Input: part model. Units: mm. Frame: model coordinates. A direction names the side the tool comes from. Coordinates: 2 decimals unless noted, no trailing zeros. Write each loop counter-clockwise with the first axis right and the second up, starting at its lowest first coordinate (ties: lowest second). Pieces come first, ordered by that corner, then holes. Notation, with made-up numbers: (54, 61) -> (75, 61) arc R30 ccw to (75, 94) -> close; hole circle Ø9 at (43.25, -26.75). An arc over 180 degrees is marked (long way). One line per question, with ' | ' between items. Start each with the question number.
```python
from build123d import *

# Parameters (mm, degrees)
F0_W     = 17
F0_H     = 2.9
F1_DEPTH = 14
F2_W     = 1.625
F2_H     = 0.32
F2_W_2   = 1
F2_H_2   = 0.58
F3_DEPTH = 12.5
F4_W     = 17
F4_H     = 1.6
F5_DEPTH = 2
F6_SIZE  = 1


with BuildPart() as f1:
    # F0 (on Top) → F1 (new body)
    with BuildSketch(Plane.XY):
        with Locations((8.5, 1.45)):
            Rectangle(F0_W, F0_H)
    extrude(amount=F1_DEPTH)

    # F2 (on face) → F3 (cut)
    with BuildSketch(Plane.XY.offset(14)):
        Polygon((15.375, 2.9), (8.5, 2.9), (1.625, 2.9), (1.625, 2.58), (1.625, 1.3), (15.375, 1.3), (15.375, 2.58), align=None)
        with Locations((16.1875, 2.74)):
            Rectangle(F2_W, F2_H)
        with Locations((0.8125, 2.74)):
            Rectangle(F2_W, F2_H)
        with Locations((16.5, 1.59)):
            Rectangle(F2_W_2, F2_H_2)
        with Locations((0.5, 1.59)):
            Rectangle(F2_W_2, F2_H_2)
    extrude(amount=-F3_DEPTH, mode=Mode.SUBTRACT)

    # F4 (on face) → F5 (cut)
    with BuildSketch(Plane.XY.offset(14)):
        with Locations((8.5, 2.1)):
            Rectangle(F4_W, F4_H)
    extrude(amount=-F5_DEPTH, mode=Mode.SUBTRACT)

    # F6
    f6_edges = [f1.edges().sort_by_distance(p)[0] for p in [
        (8.5, 0, 0),
    ]]
    chamfer(f6_edges, length=F6_SIZE)


solid = f1.part
```
1) Section A-A, the plane z = 7.75. Return loops of the section in (x, y) (3 decimals), then the cut area to 3 significant figures.
2) Section C-C, the plane y = 0.35. Return loops of the section in (x, z).
3) Ray query, line 1 (X direction, y = 1.4, z = 8.5) (3 decimals); line 2 (X direction, y = 2.5, z = 6.75) (3 decimals); line 3 (Z direction, x = 9.25, y = 1.6). Return the intervals inside material, ascending.
4) Access query for faces 4 (the face through (16, 2.58, 7)), 5 (the face through (1.625, 2, 7)), 6 (the face through (0.5, 1.88, 6.8)), 7 (the face through (8, 1, 14)), 8 (the face through (8, 0, 7)). Directions: +Z, -Z, +X, -X, +Y, -Y. A direction counts if a zero-diameter tool reaches every point of the face in a straight line with its end or side. Return the directions, or none.
5) Section B-B, the plane x = 5.5. Return loops of the section in (y, z), then the cut area to 3 significant figures.
6) Pull-direction query (Y, two-part tool) for faces 1 (the face through (17, 1, 7)), 2 (the face through (16.5, 1.88, 6.8)), 3 (the face through (8, 2.9, 1)); classes: released by +Y, released by -Y, zero draft, split by the parting line, or undercut.
7) Section D-D, the plane z = 12.5. Return loops of the section in (x, y), then the cut area to 3 significant figures.
8) First-contact query: P1, Ø1.3, axis at x = 0.5, z = 5, coming from the +Y side; P2, Ø0.8, axis at x = 12.5, y = 2.5, coming from the +Z side; P3, Ø5, axis at x = 12, z = 5, coming from the +Y side. Flat tips, straight axial feed; report the tip coordinate or a pass-through.
Answer block:
1) outline: (0, 0) -> (17, 0) -> (17, 1.3) -> (16, 1.3) -> (16, 1.88) -> (17, 1.88) -> (17, 2.58) -> (15.375, 2.58) -> (15.375, 1.3) -> (1.625, 1.3) -> (1.625, 2.58) -> (0, 2.58) -> (0, 1.88) -> (1, 1.88) -> (1, 1.3) -> (0, 1.3) -> close | area: 25.1 mm2
2) outline: (0, 0.65) -> (17, 0.65) -> (17, 14) -> (0, 14) -> close
3) line 1: x = 1 to 1.625, 15.375 to 16 | line 2: x = 0 to 1.625, 15.375 to 17 | line 3: z = 0 to 1.5
4) face 4: +Z, +X, -X, +Y | face 5: +Z, +Y | face 6: +Z, -X | face 7: +Z, +X, -X, +Y, -Y | face 8: +Z, -Z, +X, -X, -Y
5) outline: (0, 1) -> (1, 0) -> (2.9, 0) -> (2.9, 1.5) -> (1.3, 1.5) -> (1.3, 14) -> (0, 14) -> close | area: 20.1 mm2
6) face 1: zero draft | face 2: undercut | face 3: released by +Y
7) outline: (0, 0) -> (17, 0) -> (17, 1.3) -> (0, 1.3) -> close | area: 22.1 mm2
8) P1: stops at y = 2.58 | P2: stops at z = 1.5 | P3: stops at y = 1.3
